Check sheet for the modelled part. Datum: model origin and axes. Units: mm. Face numbers are marked on the shaded views. A direction names the side the tool comes from. Give positions to 0.01 mm unless a question says otherwise; leave off trailing zeros. Write each loop counter-clockwise with the first axis right and the second up, starting at its lowest first coordinate (ties: lowest second). Pieces come first, ordered by that corner, then holes. Notation, with made-up numbers: M -10.5,28 L 9.5,28 A36 ccw 9.5,64 Z; hole C -31.75,-9 d1. An arc over 180 degrees is marked long. Use CSV: the item, a comma, the result in double quotes. Start each with the question number.
1. Cross-section at B-B, the plane z = 2.5. Enter the section's corners in (x, y).
2. Cross-section at A-A, the plane x = 11.25. Enter the section's corners in (y, z).
3. Mould release check, pull along Z, two halves, no side actions. Record for the marked faces 1, 2, 3 and 4: +Z half, -Z half, draft (parallel to the pull), parting line (faces both ways), or undercut.
4. Access from +Z, -Z, +X, -X, +Y, -Y to the whole of each face (thin tool, end or side, straight path). Record for the marked faces 5 and 6.
5. Scan lines: line 1 (Y direction, x = -2, z = 1.95); line 2 (Y direction, x = 14.75, z = -0.7); line 3 (X direction, y = -2.25, z = 0.5). Record each from-to range of solid material in increasing order.
6. Cross-section at D-D, the plane z = 0.9. Enter the section's corners in (x, y), and give its area (3 significant figures).
7. Depth check by flat-ended pin: P1, Ø1.8, axis at x = 9, z = 1, coming from the -Y side. Enter the tip coordinate at first touch or a pass-through.
8. Cross-section at C-C, the plane y = 0. Enter the section's corners in (x, z), and give its area (3 significant figures).
Autodesk Inventor part; units mm, degrees
ref_plane "YZ Plane" through (0, 0, 0) normal (1, 0, 0) x (0, 1, 0)
ref_plane "XZ Plane" through (0, 0, 0) normal (0, 1, 0) x (-1, 0, 0)
ref_plane "XY Plane" through (0, 0, 0) normal (0, 0, 1) x (1, 0, 0)
sketch "Szkic1" plane through (0, 0, 0) normal (0, 0, 1) x (1, 0, 0)
  line L0 (-2.3024, 6.9387) -> (14.6976, 6.9387)
  line L1 (18.6976, 2.9387) -> (18.6976, -4.0613)
  line L2 (14.6976, -8.0613) -> (-2.3024, -8.0613)
  line L3 (-6.3024, -4.0613) -> (-6.3024, 2.9387)
  arc A0 (-2.3024, 6.9387) -> (-6.3024, 2.9387) centre (-2.3024, 2.9387) ccw
  arc A1 (18.6976, 2.9387) -> (14.6976, 6.9387) centre (14.6976, 2.9387) ccw
  arc A2 (14.6976, -8.0613) -> (18.6976, -4.0613) centre (14.6976, -4.0613) ccw
  arc A3 (-6.3024, -4.0613) -> (-2.3024, -8.0613) centre (-2.3024, -4.0613) ccw
  line L4 (14.6976, 6.4887) -> (-2.3024, 6.4887)
  arc A4 (-2.3024, 6.4887) -> (-5.8524, 2.9387) centre (-2.3024, 2.9387) ccw
  line L5 (-5.8524, 2.9387) -> (-5.8524, -4.0613)
  arc A5 (-5.8524, -4.0613) -> (-2.3024, -7.6113) centre (-2.3024, -4.0613) ccw
  line L6 (-2.3024, -7.6113) -> (14.6976, -7.6113)
  arc A6 (14.6976, -7.6113) -> (18.2476, -4.0613) centre (14.6976, -4.0613) ccw
  line L7 (18.2476, -4.0613) -> (18.2476, 2.9387)
  arc A7 (18.2476, 2.9387) -> (14.6976, 6.4887) centre (14.6976, 2.9387) ccw
  point P0 (0, 0)
  point P1 (18.6976, -8.0613)
  point P2 (18.6976, 6.9387)
  point P3 (-6.3024, -8.0613)
  dimension "d0" = 25
  dimension "d1" = 15
  dimension "d2" = 4
  dimension "d3" = 0.45
extrude "Wyciągnięcie proste1" add sketch "Szkic1" along normal blind 2.2
sketch "Szkic2" plane through (0, 0, 2.2) normal (0, 0, 1) x (1, 0, 0)
  arc A0 (18.2476, 2.9387) -> (14.6976, 6.4887) centre (14.6976, 2.9387) ccw
  line L0 (18.2476, 2.9387) -> (18.2476, -4.0613)
  arc A1 (14.6976, -7.6113) -> (18.2476, -4.0613) centre (14.6976, -4.0613) ccw
  line L1 (14.6976, -7.6113) -> (-2.3024, -7.6113)
  arc A2 (-5.8524, -4.0613) -> (-2.3024, -7.6113) centre (-2.3024, -4.0613) ccw
  line L2 (-5.8524, -4.0613) -> (-5.8524, 2.9387)
  arc A3 (-2.3024, 6.4887) -> (-5.8524, 2.9387) centre (-2.3024, 2.9387) ccw
  line L3 (-2.3024, 6.4887) -> (14.6976, 6.4887)
  line L4 (-6.3024, 2.9387) -> (-6.3024, -4.0613)
  arc A4 (-6.3024, -4.0613) -> (-2.3024, -8.0613) centre (-2.3024, -4.0613) ccw
  line L5 (-2.3024, -8.0613) -> (14.6976, -8.0613)
  arc A5 (14.6976, -8.0613) -> (18.6976, -4.0613) centre (14.6976, -4.0613) ccw
  line L6 (18.6976, -4.0613) -> (18.6976, 2.9387)
  arc A6 (18.6976, 2.9387) -> (14.6976, 6.9387) centre (14.6976, 2.9387) ccw
  line L7 (14.6976, 6.9387) -> (-2.3024, 6.9387)
  arc A7 (-2.3024, 6.9387) -> (-6.3024, 2.9387) centre (-2.3024, 2.9387) ccw
  line L8 (-7.3024, 2.9387) -> (-7.3024, -4.0613)
  arc A8 (-7.3024, -4.0613) -> (-2.3024, -9.0613) centre (-2.3024, -4.0613) ccw
  line L9 (-2.3024, -9.0613) -> (14.6976, -9.0613)
  arc A9 (14.6976, -9.0613) -> (19.6976, -4.0613) centre (14.6976, -4.0613) ccw
  line L10 (19.6976, -4.0613) -> (19.6976, 2.9387)
  arc A10 (19.6976, 2.9387) -> (14.6976, 7.9387) centre (14.6976, 2.9387) ccw
  line L11 (14.6976, 7.9387) -> (-2.3024, 7.9387)
  arc A11 (-2.3024, 7.9387) -> (-7.3024, 2.9387) centre (-2.3024, 2.9387) ccw
  point P0 (0, 0)
  dimension "d6" = 1
extrude "Wyciągnięcie proste2" add sketch "Szkic2" along normal blind 1 contours A7 L7 A6 L6 A5 L5 A4 L4 | A11 L11 A10 L10 A9 L9 A8 L8
sketch "Szkic3" plane through (0, 0, 0) normal (0, 0, -1) x (-1, 0, 0)
  line L0 (7.3024, 2.9387) -> (7.3024, -4.0613)
  arc A0 (7.3024, 2.9387) -> (2.3024, 7.9387) centre (2.3024, 2.9387) ccw
  line L1 (-14.6976, 7.9387) -> (2.3024, 7.9387)
  arc A1 (-14.6976, 7.9387) -> (-19.6976, 2.9387) centre (-14.6976, 2.9387) ccw
  line L2 (-19.6976, -4.0613) -> (-19.6976, 2.9387)
  arc A2 (-19.6976, -4.0613) -> (-14.6976, -9.0613) centre (-14.6976, -4.0613) ccw
  line L3 (2.3024, -9.0613) -> (-14.6976, -9.0613)
  arc A3 (2.3024, -9.0613) -> (7.3024, -4.0613) centre (2.3024, -4.0613) ccw
  arc A4 (6.3024, 2.9387) -> (2.3024, 6.9387) centre (2.3024, 2.9387) ccw
  line L4 (6.3024, 2.9387) -> (6.3024, -4.0613)
  arc A5 (2.3024, -8.0613) -> (6.3024, -4.0613) centre (2.3024, -4.0613) ccw
  line L5 (2.3024, -8.0613) -> (-14.6976, -8.0613)
  arc A6 (-18.6976, -4.0613) -> (-14.6976, -8.0613) centre (-14.6976, -4.0613) ccw
  line L6 (-18.6976, -4.0613) -> (-18.6976, 2.9387)
  arc A7 (-14.6976, 6.9387) -> (-18.6976, 2.9387) centre (-14.6976, 2.9387) ccw
  line L7 (-14.6976, 6.9387) -> (2.3024, 6.9387)
  arc A8 (-14.6976, 6.4887) -> (-18.2476, 2.9387) centre (-14.6976, 2.9387) ccw
  line L8 (-14.6976, 6.4887) -> (2.3024, 6.4887)
  arc A9 (5.8524, 2.9387) -> (2.3024, 6.4887) centre (2.3024, 2.9387) ccw
  line L9 (5.8524, 2.9387) -> (5.8524, -4.0613)
  arc A10 (2.3024, -7.6113) -> (5.8524, -4.0613) centre (2.3024, -4.0613) ccw
  line L10 (2.3024, -7.6113) -> (-14.6976, -7.6113)
  arc A11 (-18.2476, -4.0613) -> (-14.6976, -7.6113) centre (-14.6976, -4.0613) ccw
  line L11 (-18.2476, -4.0613) -> (-18.2476, 2.9387)
  line L12 (6.3024, 2.9387) -> (6.3024, -4.0613)
  arc A12 (6.3024, 2.9387) -> (2.3024, 6.9387) centre (2.3024, 2.9387) ccw
  line L13 (-14.6976, 6.9387) -> (2.3024, 6.9387)
  arc A13 (-14.6976, 6.9387) -> (-18.6976, 2.9387) centre (-14.6976, 2.9387) ccw
  line L14 (-18.6976, -4.0613) -> (-18.6976, 2.9387)
  arc A14 (-18.6976, -4.0613) -> (-14.6976, -8.0613) centre (-14.6976, -4.0613) ccw
  line L15 (2.3024, -8.0613) -> (-14.6976, -8.0613)
  arc A15 (2.3024, -8.0613) -> (6.3024, -4.0613) centre (2.3024, -4.0613) ccw
  point P0 (0, 0)
extrude "Wyciągnięcie proste3" add sketch "Szkic3" along normal blind 1 contours L0 A3 L3 A2 L2 A1 L1 A0 | L4 A5 L5 A6 L6 A7 L7 A4
properties part number "3DP_TPU_Cable_Feed_Through_25mm"
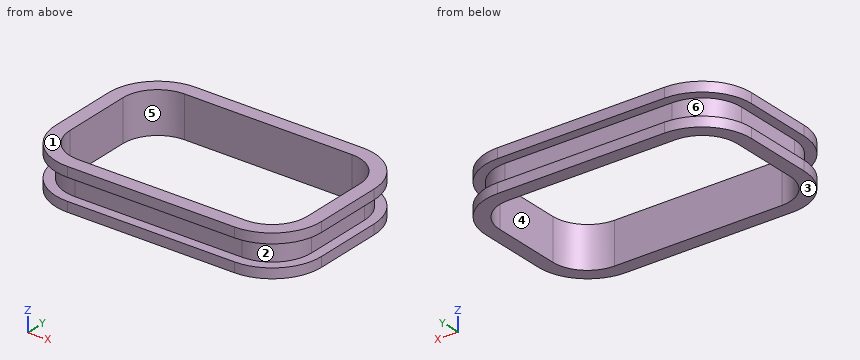
Worked answers:
1,outline,"M -7.3,-4.06 A5 ccw -2.3,-9.06 L 14.7,-9.06 A5 ccw 19.7,-4.06 L 19.7,2.94 A5 ccw 14.7,7.94 L -2.3,7.94 A5 ccw -7.3,2.94 Z; hole M -5.85,-4.06 A3.55 ccw -2.3,-7.61 L 14.7,-7.61 A3.55 ccw 18.25,-4.06 L 18.25,2.94 A3.55 ccw 14.7,6.49 L -2.3,6.49 A3.55 ccw -5.85,2.94 Z"
2,outline,"M -9.06,-1 L -7.61,-1 L -7.61,3.2 L -9.06,3.2 L -9.06,2.2 L -8.06,2.2 L -8.06,0 L -9.06,0 Z; M 6.49,-1 L 7.94,-1 L 7.94,0 L 6.94,0 L 6.94,2.2 L 7.94,2.2 L 7.94,3.2 L 6.49,3.2 Z"
3,face 1,"+Z half"
3,face 2,"undercut"
3,face 3,"-Z half"
3,face 4,"draft"
4,face 5,"+Z, -Z"
4,face 6,"-X, +Y"
5,line 1,"y = -8.06 to -7.61, 6.49 to 6.94"
5,line 2,"y = -9.06 to -7.61, 6.49 to 7.94"
5,line 3,"x = -6.3 to -5.85, 18.25 to 18.7"
6,outline,"M -6.3,-4.06 A4 ccw -2.3,-8.06 L 14.7,-8.06 A4 ccw 18.7,-4.06 L 18.7,2.94 A4 ccw 14.7,6.94 L -2.3,6.94 A4 ccw -6.3,2.94 Z; hole M -5.85,-4.06 A3.55 ccw -2.3,-7.61 L 14.7,-7.61 A3.55 ccw 18.25,-4.06 L 18.25,2.94 A3.55 ccw 14.7,6.49 L -2.3,6.49 A3.55 ccw -5.85,2.94 Z"
6,area,"32.3 mm^2"
7,P1,"stops at y = -8.06"
8,outline,"M -7.3,-1 L -5.85,-1 L -5.85,3.2 L -7.3,3.2 L -7.3,2.2 L -6.3,2.2 L -6.3,0 L -7.3,0 Z; M 18.25,-1 L 19.7,-1 L 19.7,0 L 18.7,0 L 18.7,2.2 L 19.7,2.2 L 19.7,3.2 L 18.25,3.2 Z"
8,area,"7.78 mm^2"
